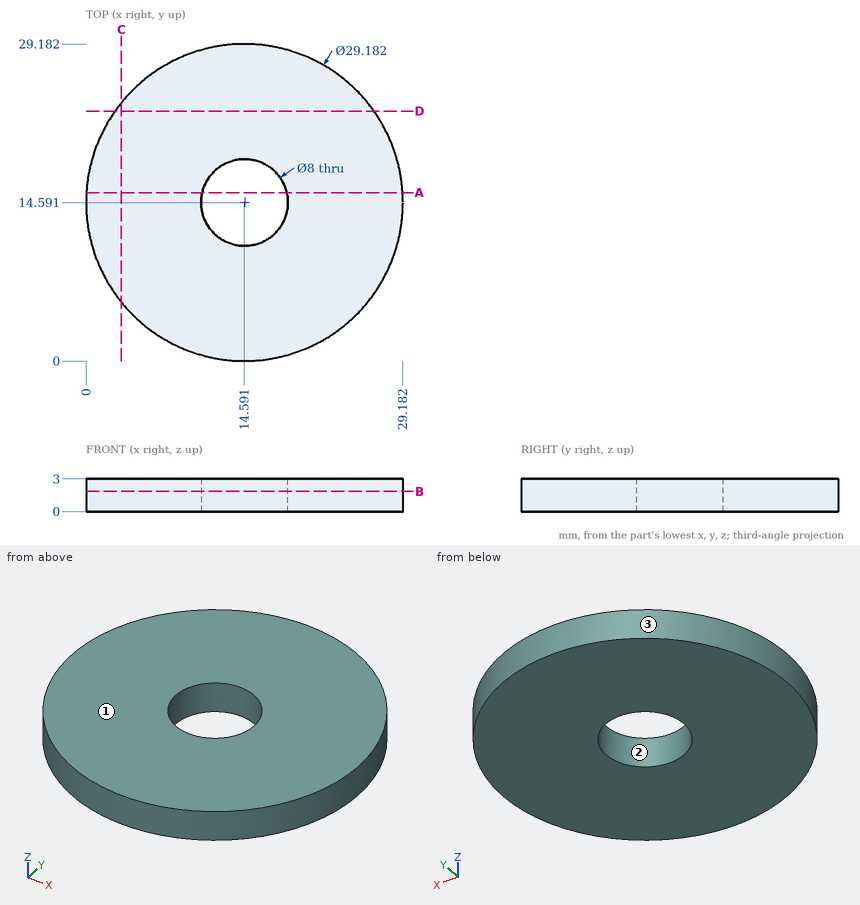
For this review, use the dimensioned drawing (mm, ordinates from the lowest corner) and the shaded views. Round coordinates to 2 decimals unless told otherwise and drop trailing zeros. Write each loop counter-clockwise with the first axis right and the second up, starting at its lowest first coordinate (ties: lowest second). Pieces come first, ordered by that corner, then holes. Notation, with made-up numbers: M 17.25,72.25 L 68.25,72.25 A24 cw 68.25,88.25 Z; hole C 41.25,-12.5 d2. An arc over 180 degrees is marked long. Write item = value, one per line. Start each with the question number.
(1) For line 1 along X through (y, z) = (16.75, 0.6); line 2 along X through (y, z) = (18, 1.2) (1 decimal); line 3 along Y through (x, z) = (14.25, 2.3), list the stretches that pass through material, from the lowest coordinate up.
(2) We need section D-D (y = 23). Give the boundary of the cut face in (x, z).
(3) We need section C-C (x = 3.25). Give the boundary of the cut face in (y, z), then the cut area to 3 significant figures.
(4) The part is to be moulded in two halves that separate along Y. For the marked faces 1, 2 and 3, say which applies: +Y half, -Y half, draft (parallel to the pull), parting line (faces both ways), or undercut.
(5) We need section B-B (z = 1.85). Give the boundary of the cut face in (x, y).
(6) Clearance check with a flat-ended pin moving along its axis: pin 1 Ø1 at (x, z) = (8.5, 1) entering from +Y. State where the tip first meets the part, or that it passes through.
(7) We need section A-A (y = 15.5). Give the boundary of the cut face in (x, z), then the cut area to 3 significant figures.
Results found:
q1.line_1 = 0.16 to 11.22, 17.96 to 29.02
q1.line_2 = 0.4 to 12.5, 16.7 to 28.8
q1.line_3 = 0 to 10.61, 18.58 to 29.18
q2.outline = M 2.67,0 L 26.52,0 L 26.52,3 L 2.67,3 Z
q3.outline = M 5.41,0 L 23.77,0 L 23.77,3 L 5.41,3 Z
q3.area = 55.1 mm²
q4.face_1 = draft
q4.face_2 = undercut
q4.face_3 = parting line
q5.outline = C 14.59,14.59 d29.18; hole C 14.59,14.59 d8
q6.pin_1 = 28.07
q7.outline = M 0.03,0 L 10.7,0 L 10.7,3 L 0.03,3 Z; M 18.49,0 L 29.15,0 L 29.15,3 L 18.49,3 Z
q7.area = 64.0 mm²
